Design review of the part built by this model. Coordinates are the model's own, in mm. A direction names the side the tool comes from. Coordinates: 2 decimals unless noted, no trailing zeros. Order: outer loops, then holes, each group sorted by start corner. A loop starts at its lowest first (then second) coordinate and runs counter-clockwise, first axis right, second up. Notation, with made-up numbers: M 33.25,76.5 L 48.25,76.5 A24 ccw 48.25,91.5 Z; hole C 54.25,81 d3. An arc over 180 degrees is marked long. Answer as a JSON object with one key per item and string values.
Autodesk Inventor part; units mm, degrees
ref_plane "YZ Plane" through (0, 0, 0) normal (1, 0, 0) x (0, 1, 0)
ref_plane "XZ Plane" through (0, 0, 0) normal (0, 1, 0) x (-1, 0, 0)
ref_plane "XY Plane" through (0, 0, 0) normal (0, 0, 1) x (1, 0, 0)
sketch "Sketch1" plane through (0, 0, 0) normal (0, 0, 1) x (1, 0, 0)
  line L0 (-20, -20) -> (20, -20)
  line L1 (20, -20) -> (20, 20)
  line L2 (20, 20) -> (-20, 20)
  line L3 (-20, 20) -> (-20, -20)
  line L4 (-20, -20) -> (20, 20) construction
  line L5 (20, -20) -> (-20, 20) construction
  circle A0 centre (0, 0) radius 15.875
  dimension "d0" = 40
  dimension "d51" = 31.75
extrude "Extrusion1" add sketch "Sketch1" along normal blind 2 contours A0
sketch "Sketch10" plane through (0, 0, 2) normal (0, 0, 1) x (1, 0, 0)
  circle A0 centre (0, 0) radius 10
  dimension "d64" = 20
extrude "Extrusion8" add sketch "Sketch10" along normal blind 100
sketch "Sketch4" plane through (0, 0, 102) normal (0, 0, 1) x (1, 0, 0)
  line L0 (-4, 4) -> (4, 4)
  line L1 (4, 4) -> (4, -4)
  line L2 (4, -4) -> (-4, -4)
  line L3 (-4, -4) -> (-4, 4)
  line L4 (-4, 4) -> (4, -4) construction
  line L5 (4, 4) -> (-4, -4) construction
  line L6 (4, -1) -> (5, -1)
  line L7 (5, -1) -> (5, -5)
  line L8 (5, -5) -> (1, -5)
  line L9 (1, -5) -> (1, -4)
  point P0 (0, 0)
  point P1 (0, 0)
  point P2 (0, 0)
  point P3 (-5, 5)
  point P4 (0, 0)
  dimension "d16" = 8
  dimension "d17" = 1
  dimension "d18" = 4
  dimension "d30" = 5
  dimension "d31" = 5
sketch "Sketch9" plane through (0, 0, 0) normal (0, 0, -1) x (-1, 0, 0)
  circle A0 centre (0, 0) radius 12.7
  dimension "d52" = 25.4
extrude "Extrusion6" add sketch "Sketch9" along normal blind 10
extrude "Extrusion7" add sketch "Sketch4" along normal blind 1 contours L6 L7 L8 L9 L2 L1
hole "Hole4" at (-5, 5, 102) direction (0, 0, -1) diameter 1.425 depth 5.692 tip angle 118
properties part number "ChipMount"
1) Insertion check: pin 1 Ø10 at (x, z) = (-2.5, 45.5) entering from +Y; pin 2 Ø12 at (x, z) = (3, 71.5) entering from -Y; pin 3 Ø6 at (y, z) = (-4, 51.5) entering from +X. Each pin has a flat end and moves straight along its axis. Give the tip position at first contact, or say it passes through.
Taken from the geometry:
{"pin 1": "stops at y = 10", "pin 2": "stops at y = -10", "pin 3": "stops at x = 9.95"}
2) Add section C-C (z = 14). State the section outline as (x, y) points, and give its area (3 significant figures).
Taken from the geometry:
{"outline": "C 0,0 d20", "area": "314 mm2"}
3) Tool access review of faces 1 (the flat face through (-7, 11, 0)), 2 (the flat face through (4.3, -3.9, 103)), 3 (the cylindrical face through (-2.17, 9.76, 51.3)): name each direction out of +Z, -Z, +X, -X, +Y, -Y from which nothing blocks a thin tool from reaching the whole face with its end or side.
Taken from the geometry:
{"face 1": "-Z", "face 2": "+Z, +X, -X, +Y, -Y", "face 3": "+Z"}
4) Add section A-A (y = 0). State the section outline as (x, z) points (3 decimals), and give its area (3 significant figures).
Taken from the geometry:
{"outline": "M -15.875,0 L -12.7,0 L -12.7,-10 L 12.7,-10 L 12.7,0 L 15.875,0 L 15.875,2 L 10,2 L 10,102 L -10,102 L -10,2 L -15.875,2 Z", "area": "2,320 mm2"}
5) To check wall thickness, follow L1, parallel to Z at x = 7, y = 12; L2, parallel to X at y = 5, z = 98.9; L3, parallel to Z at x = -9, y = -8. State the ranges of each line that lie inside material, in increasing order.
Taken from the geometry:
{"L1": "z = 0 to 2", "L2": "x = -8.66 to -5.71, -4.29 to 8.66", "L3": "z = -10 to 2"}
